Can you work these out from the model? Positions are in its coordinate system, mm. A direction names the side the tool comes from. Round coordinates to 2 decimals unless told otherwise and drop trailing zeros. Loops run counter-clockwise (first coordinate to the right, second up) from the corner with the lowest first, then second, coordinate; pieces in that order, holes last. Notation, with made-up numbers: (86.25, 62) - (144.25, 62) arc R24 ccw to (144.25, 94) - close; hole circle Ø9 at (38.5, 4). An arc over 180 degrees is marked (long way). Answer as CSV lines item,"result".
```python
from build123d import *

# Parameters (mm, degrees)
F0_W     = 120
F0_H     = 60
F1_DEPTH = 175
F2_T     = -2
F3_R     = 5
F4_R     = 4.5
F5_DEPTH = 60.001


with BuildPart() as f1:
    # F0 (on Top) → F1 (new body, symmetric)
    with BuildSketch(Plane.XY):
        Rectangle(F0_W, F0_H)
    extrude(amount=F1_DEPTH, both=True)

    # F2
    f2_openings = [f1.faces().sort_by_distance(p)[0] for p in [
        (0, 30, 0),
        (0, 0, 175),
        (0, 0, -175),
    ]]
    offset(amount=F2_T, openings=f2_openings)

    # F3
    f3_edges = [f1.edges().sort_by_distance(p)[0] for p in [
        (60, -30, 0),
        (-58, -28, 0),
        (58, -28, 0),
        (-60, -30, 0),
    ]]
    fillet(f3_edges, radius=F3_R)

    # F4 (on face) → F5 (cut, through all)
    with BuildSketch(Plane.XZ.offset(30)):
        Circle(F4_R)
    extrude(amount=-F5_DEPTH, mode=Mode.SUBTRACT)


solid = f1.part
```
Q1. Imagine slicing it at C-C (y = 25). Write out the boundary of the cut face in (x, z), then the cut area to 3 significant figures.
Checks:
outline,"(-60, -175) - (-58, -175) - (-58, 175) - (-60, 175) - close; (58, -175) - (60, -175) - (60, 175) - (58, 175) - close"
area,"1,400 mm²"
Q2. Imagine slicing it at A-A (x = 0). Write out the boundary of the cut face in (y, z).
Checks:
outline,"(-30, -175) - (-28, -175) - (-28, -4.5) - (-30, -4.5) - close; (-30, 4.5) - (-28, 4.5) - (-28, 175) - (-30, 175) - close"
Q3. Imagine slicing it at D-D (z = 69.5). Write out the boundary of the cut face in (x, y), then the cut area to 3 significant figures.
Checks:
outline,"(-60, -25) arc R5 ccw to (-55, -30) - (55, -30) arc R5 ccw to (60, -25) - (60, 30) - (58, 30) - (58, -23) arc R5 cw to (53, -28) - (-53, -28) arc R5 cw to (-58, -23) - (-58, 30) - (-60, 30) - close"
area,"472 mm²"
Q4. On a 3-axis mill with a long thin cutter (end or side, diameter ignored), from which of +Z, -Z, +X, -X, +Y, -Y can I reach the whole of each face in a straight line? I mean faces 1 (the flat face through (11, -28, 2)), 2 (the flat face through (-13, -30, 2)). Say none if no direction works.
Checks:
face 1,"+Z, -Z, +Y"
face 2,"+Z, -Z, +X, -X, -Y"
Q5. We'd pull the mould along Z, two halves only. Please class faces 3 (the flat face through (-27, -29, -175)), 4 (the flat face through (60, 2, 2)), 5 (the cylindrical face through (-0.59, -29.01, 4.46)): pulls with the +Z half, pulls with the -Z half, needs draft (parallel to the pull), parting line crosses it, or undercut.
Checks:
face 3,"pulls with the -Z half"
face 4,"needs draft"
face 5,"undercut"
Q6. If I drill on line 1 along X through (y, z) = (9.5, -55.5); line 2 along Z through (x, y) = (0, -29.35); line 3 along Y through (x, z) = (15.5, 99), over which ranges is the centre line in solid material (lowest first)? Write a range as [from, to].
Checks:
line 1,"[-60, -58], [58, 60]"
line 2,"[-175, -4.5], [4.5, 175]"
line 3,"[-30, -28]"
Q7. I'm going to push flat-ended pins straight in: pin 1 Ø10.5 at (x, z) = (0, 0) entering from -Y; pin 2 Ø10 at (x, z) = (-38.5, 5) entering from +Y. Where does each tip first touch, or does it pass through?
Checks:
pin 1,"y = -30"
pin 2,"y = -28"
Q8. Imagine slicing it at B-B (z = 0). Write out the boundary of the cut face in (x, y), then the cut area to 3 significant figures.
Checks:
outline,"(-60, -25) arc R5 ccw to (-55, -30) - (-4.5, -30) - (-4.5, -28) - (-53, -28) arc R5 cw to (-58, -23) - (-58, 30) - (-60, 30) - close; (4.5, -30) - (55, -30) arc R5 ccw to (60, -25) - (60, 30) - (58, 30) - (58, -23) arc R5 cw to (53, -28) - (4.5, -28) - close"
area,"454 mm²"
